Read the model definition and answer for the solid it produces. Units are mm, in the model's axes. Give positions to 0.01 mm unless a question says otherwise; leave off trailing zeros. Write each loop counter-clockwise with the first axis right and the second up, starting at its lowest first coordinate (ties: lowest second). Pieces come first, ordered by that corner, then holes. Notation, with made-up numbers: M 27,-16 L 83,-16 A35 cw 83,23 Z; hole C 58.25,54.25 d10. An arc over 180 degrees is marked long. Put each result on its own line as item: value.
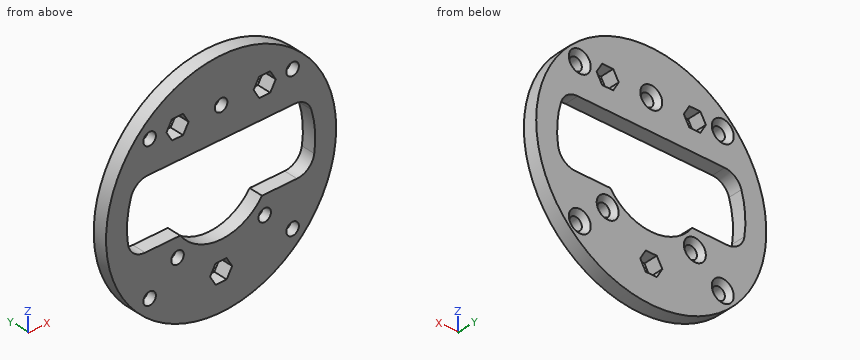
from build123d import *

# Parameters (mm, degrees)
SKETCH1_R                                       = 33
SKETCH1_R_2                                     = 27
BOSS_EXTRUDE1_DEPTH                             = 4
SKETCH2_R                                       = 1.5
SALIENTE_EXTRUIR1_DEPTH                         = 4
CORTAR_EXTRUIR1_REACH                           = 6
CROQUIS1_R                                      = 1.75
CSK_FOR_M3_FLAT_HEAD_MACHINE_SCREW1_D           = 3.6
CSK_FOR_M3_FLAT_HEAD_MACHINE_SCREW1_CSINK_D     = 6.3
CSK_FOR_M3_FLAT_HEAD_MACHINE_SCREW1_CSINK_ANGLE = 90
CSK_FOR_M3_FLAT_HEAD_MACHINE_SCREW2_D           = 3.6
CSK_FOR_M3_FLAT_HEAD_MACHINE_SCREW2_CSINK_D     = 6.3
CSK_FOR_M3_FLAT_HEAD_MACHINE_SCREW2_CSINK_ANGLE = 90
FILLET1_R                                       = 5


with BuildPart() as part:
    # Sketch1 → Boss-Extrude1 (new body)
    with BuildSketch(Plane(origin=(0, 0, 0), x_dir=(1, 0, 0), z_dir=(0, 1, 0))):
        Circle(SKETCH1_R)
        Circle(SKETCH1_R_2, mode=Mode.SUBTRACT)
    extrude(amount=BOSS_EXTRUDE1_DEPTH)

    # Sketch2 → Saliente-Extruir1 (add)
    with BuildSketch(Plane(origin=(0, 4, 0), x_dir=(1, 0, 0), z_dir=(0, 1, 0))):
        with BuildLine():
            Line((-24.5, -11.346805718), (24.5, -11.346805718))
            ThreePointArc((24.5, -11.346805718), (0, -27), (-24.5, -11.346805718))
        make_face()
        with Locations((0, -20.2)):
            Circle(SKETCH2_R, mode=Mode.SUBTRACT)
        with BuildLine():
            Line((-25.7325, 8.175478197), (-11.7325, 8.175478197))
            ThreePointArc((-11.7325, 8.175478197), (0, 14.3), (11.7325, 8.175478197))
            Line((11.7325, 8.175478197), (25.7325, 8.175478197))
            ThreePointArc((25.7325, 8.175478197), (0, 27), (-25.7325, 8.175478197))
        make_face()
        with Locations((-12.5, 13.5)):
            Circle(SKETCH2_R, mode=Mode.SUBTRACT)
        with Locations((12.5, 13.5)):
            Circle(SKETCH2_R, mode=Mode.SUBTRACT)
    extrude(amount=-SALIENTE_EXTRUIR1_DEPTH)

    # Croquis1 → Cortar-Extruir1 (cut, up to next)
    with BuildSketch(Plane(origin=(0, 4, 0), x_dir=(1, 0, 0), z_dir=(0, 1, 0)), mode=Mode.PRIVATE) as cortar_extruir1_sk1:
        with Locations((-20.506096654, 20.506096654)):
            Circle(CROQUIS1_R)
    cortar_extruir1_tool1 = extrude(cortar_extruir1_sk1.sketch, amount=-CORTAR_EXTRUIR1_REACH, mode=Mode.PRIVATE) & part.part
    add(cortar_extruir1_tool1.solids().sort_by_distance((-20.506097, 4, -20.506097))[0], mode=Mode.SUBTRACT)
    # Croquis1 → Cortar-Extruir1 (cut, up to next)
    with BuildSketch(Plane(origin=(0, 4, 0), x_dir=(1, 0, 0), z_dir=(0, 1, 0)), mode=Mode.PRIVATE) as cortar_extruir1_sk2:
        with Locations((20.506096654, 20.506096654)):
            Circle(CROQUIS1_R)
    cortar_extruir1_tool2 = extrude(cortar_extruir1_sk2.sketch, amount=-CORTAR_EXTRUIR1_REACH, mode=Mode.PRIVATE) & part.part
    add(cortar_extruir1_tool2.solids().sort_by_distance((20.506097, 4, -20.506097))[0], mode=Mode.SUBTRACT)
    # Croquis1 → Cortar-Extruir1 (cut, up to next)
    with BuildSketch(Plane(origin=(0, 4, 0), x_dir=(1, 0, 0), z_dir=(0, 1, 0)), mode=Mode.PRIVATE) as cortar_extruir1_sk3:
        with Locations((-20.506096654, -20.506096654)):
            Circle(CROQUIS1_R)
    cortar_extruir1_tool3 = extrude(cortar_extruir1_sk3.sketch, amount=-CORTAR_EXTRUIR1_REACH, mode=Mode.PRIVATE) & part.part
    add(cortar_extruir1_tool3.solids().sort_by_distance((-20.506097, 4, 20.506097))[0], mode=Mode.SUBTRACT)
    # Croquis1 → Cortar-Extruir1 (cut, up to next)
    with BuildSketch(Plane(origin=(0, 4, 0), x_dir=(1, 0, 0), z_dir=(0, 1, 0)), mode=Mode.PRIVATE) as cortar_extruir1_sk4:
        with Locations((20.506096654, -20.506096654)):
            Circle(CROQUIS1_R)
    cortar_extruir1_tool4 = extrude(cortar_extruir1_sk4.sketch, amount=-CORTAR_EXTRUIR1_REACH, mode=Mode.PRIVATE) & part.part
    add(cortar_extruir1_tool4.solids().sort_by_distance((20.506097, 4, 20.506097))[0], mode=Mode.SUBTRACT)
    # Croquis1 → Cortar-Extruir1 (cut, up to next)
    with BuildSketch(Plane(origin=(0, 4, 0), x_dir=(1, 0, 0), z_dir=(0, 1, 0)), mode=Mode.PRIVATE) as cortar_extruir1_sk5:
        Polygon((-9.324573519, -20), (-10.91228676, -17.25), (-14.08771324, -17.25), (-15.675426481, -20), (-14.08771324, -22.75), (-10.91228676, -22.75), align=None)
    cortar_extruir1_tool5 = extrude(cortar_extruir1_sk5.sketch, amount=-CORTAR_EXTRUIR1_REACH, mode=Mode.PRIVATE) & part.part
    add(cortar_extruir1_tool5.solids().sort_by_distance((-12.5, 4, 20))[0], mode=Mode.SUBTRACT)
    # Croquis1 → Cortar-Extruir1 (cut, up to next)
    with BuildSketch(Plane(origin=(0, 4, 0), x_dir=(1, 0, 0), z_dir=(0, 1, 0)), mode=Mode.PRIVATE) as cortar_extruir1_sk6:
        Polygon((15.675426481, -20), (14.08771324, -17.25), (10.91228676, -17.25), (9.324573519, -20), (10.91228676, -22.75), (14.08771324, -22.75), align=None)
    cortar_extruir1_tool6 = extrude(cortar_extruir1_sk6.sketch, amount=-CORTAR_EXTRUIR1_REACH, mode=Mode.PRIVATE) & part.part
    add(cortar_extruir1_tool6.solids().sort_by_distance((12.5, 4, 20))[0], mode=Mode.SUBTRACT)
    # Croquis1 → Cortar-Extruir1 (cut, up to next)
    with BuildSketch(Plane(origin=(0, 4, 0), x_dir=(1, 0, 0), z_dir=(0, 1, 0)), mode=Mode.PRIVATE) as cortar_extruir1_sk7:
        Polygon((3.175426481, 22.5), (1.58771324, 25.25), (-1.58771324, 25.25), (-3.175426481, 22.5), (-1.58771324, 19.75), (1.58771324, 19.75), align=None)
    cortar_extruir1_tool7 = extrude(cortar_extruir1_sk7.sketch, amount=-CORTAR_EXTRUIR1_REACH, mode=Mode.PRIVATE) & part.part
    add(cortar_extruir1_tool7.solids().sort_by_distance((0, 4, -22.5))[0], mode=Mode.SUBTRACT)

    # CSK for M3 Flat Head Machine Screw1 (through all)
    with Locations(Plane(origin=(0, 4, 0), x_dir=(1, 0, 0), z_dir=(0, 1, 0))):
        with Locations((-20.506096654, 20.506096654), (20.506096654, 20.506096654), (20.506096654, -20.506096654), (-20.506096654, -20.506096654)):
            CounterSinkHole(CSK_FOR_M3_FLAT_HEAD_MACHINE_SCREW1_D / 2, CSK_FOR_M3_FLAT_HEAD_MACHINE_SCREW1_CSINK_D / 2, counter_sink_angle=CSK_FOR_M3_FLAT_HEAD_MACHINE_SCREW1_CSINK_ANGLE)

    # CSK for M3 Flat Head Machine Screw2 (through all)
    with Locations(Plane(origin=(0, 4, 0), x_dir=(1, 0, 0), z_dir=(0, 1, 0))):
        with Locations((-12.5, 13.5), (12.5, 13.5), (0, -20.2)):
            CounterSinkHole(CSK_FOR_M3_FLAT_HEAD_MACHINE_SCREW2_D / 2, CSK_FOR_M3_FLAT_HEAD_MACHINE_SCREW2_CSINK_D / 2, counter_sink_angle=CSK_FOR_M3_FLAT_HEAD_MACHINE_SCREW2_CSINK_ANGLE)

    # Fillet1
    fillet1_edges = [part.edges().sort_by_distance(p)[0] for p in [
        (-25.7325, 2, -8.175478197),
        (25.7325, 2, -8.175478197),
        (24.5, 2, 11.346805718),
        (-24.5, 2, 11.346805718),
    ]]
    fillet(fillet1_edges, radius=FILLET1_R)


solid = part.part
(1) Section D-D on x = 12.5 is taken. Determine the outline of the cut face in (y, z).
Result:
outline: M 0,-30.54 L 4,-30.54 L 4,-16.65 L 2.65,-15.3 L 0,-15.3 Z; M 0,-11.7 L 2.65,-11.7 L 4,-10.35 L 4,-8.18 L 0,-8.18 Z; M 0,11.35 L 4,11.35 L 4,17.25 L 0,17.25 Z; M 0,22.75 L 4,22.75 L 4,30.54 L 0,30.54 Z
(2) Straight lines are drawn through the part: line 1 along X through (y, z) = (3.4, 0); line 2 along Z through (x, y) = (12.5, 1.05); line 3 along X through (y, z) = (2.1, -22). For each, find the intervals that lie inside material, in ascending order. Write a range as from..to.
Result:
line 1: x = -33..-27, 27..33
line 2: z = -30.54..-15.3, -11.7..-8.18, 11.35..17.25, 22.75..30.54
line 3: x = -24.6..-21.51, -19.5..-2.89, 2.89..19.5, 21.51..24.6
(3) Given pin 1 Ø1.6 at (x, y) = (0, 2.5) entering from -Z; pin 2 Ø1 at (x, y) = (0, 1.5) entering from +Z; pin 3 Ø2 at (x, y) = (-3.5, 2) entering from -Z, each flat-ended and moving along its own axis, determine where each tip first touches the part or whether it passes through.
Result:
pin 1: stops at z = -33
pin 2: stops at z = 33
pin 3: stops at z = -32.91
(4) Section C-C on z = -13.5 is taken. Determine the outline of the cut face in (x, y).
Result:
outline: M -30.11,0 L -14.3,0 L -14.3,2.65 L -15.65,4 L -30.11,4 Z; M -10.7,0 L -4.72,0 L -4.72,4 L -9.35,4 L -10.7,2.65 Z; M 4.72,0 L 10.7,0 L 10.7,2.65 L 9.35,4 L 4.72,4 Z; M 14.3,0 L 30.11,0 L 30.11,4 L 15.65,4 L 14.3,2.65 Z
(5) Section B-B on z = 0 is taken. Determine the outline of the cut face in (x, y), and give its area (3 significant figures).
Result:
outline: M -33,0 L -27,0 L -27,4 L -33,4 Z; M 27,0 L 33,0 L 33,4 L 27,4 Z
area: 48.0 mm²
(6) Section A-A on x = 0 is taken. Determine the outline of the cut face in (y, z), and give its area (3 significant figures).
Result:
outline: M 0,-33 L 4,-33 L 4,-25.25 L 0,-25.25 Z; M 0,-19.75 L 4,-19.75 L 4,-14.3 L 0,-14.3 Z; M 0,11.35 L 4,11.35 L 4,17.05 L 2.65,18.4 L 0,18.4 Z; M 0,22 L 2.65,22 L 4,23.35 L 4,33 L 0,33 Z
area: 123 mm²
